CAD build for the part. Positions are in the model's coordinates, mm. Give positions to 0.01 mm unless a question says otherwise; leave off trailing zeros. Loops run counter-clockwise (first coordinate to the right, second up) from the corner with the lowest first, then second, coordinate; pieces in that order, holes last. Notation, with made-up numbers: M 13,27.25 L 53,27.25 A26 ccw 53,52.25 Z; hole C -37,-9 d2. An arc over 180 degrees is marked long. Answer as CSV lines item,"result".
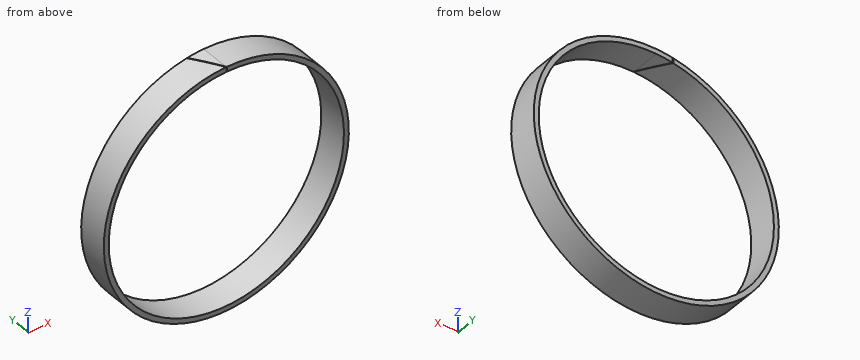
```python
from build123d import *

# Parameters (mm, degrees)
SKETCH1_R           = 25
SKETCH1_R_2         = 24
BOSS_EXTRUDE1_DEPTH = 6
CUT_EXTRUDE1_REACH  = 37.861


with BuildPart() as part:
    # Sketch1 → Boss-Extrude1 (new body)
    with BuildSketch(Plane(origin=(0, 0, 0), x_dir=(1, 0, 0), z_dir=(0, 1, 0))):
        with Locations(Location((0, 0, 0), (0, 0, 270))):
            Circle(SKETCH1_R)
        with Locations(Location((0, 0, 0), (0, 0, 270))):
            Circle(SKETCH1_R_2, mode=Mode.SUBTRACT)
    extrude(amount=BOSS_EXTRUDE1_DEPTH)

    # Sketch2 → Cut-Extrude1 (cut, up to next)
    with BuildSketch(Plane.XY, mode=Mode.PRIVATE) as cut_extrude1_sk1:
        Polygon((0, 0), (-3.464101615, 6), (-3.348631561, 6), (0.115470054, 0), align=None)
    cut_extrude1_tool1 = extrude(cut_extrude1_sk1.sketch, amount=CUT_EXTRUDE1_REACH, mode=Mode.PRIVATE) & part.part
    add(cut_extrude1_tool1.solids().sort_by_distance((-1.674316, 3, 0))[0], mode=Mode.SUBTRACT)


solid = part.part
```
Q1. Wall check: line 1 (Z direction, x = 0, y = 2.75); line 2 (Z direction, x = 6, y = 5.5). Give the ranges that are in metal, low to high. Write a range as [from, to].
Solution:
line 1,"z = [-25, -24], [24, 25]"
line 2,"z = [-24.27, -23.24], [23.24, 24.27]"
Q2. Cut at C-C (y = 4). Write the cut outline in (x, z), and give its area (3 significant figures).
Solution:
outline,"M -2.31,23.89 L -2.31,24.89 A25 ccw long -2.19,24.9 L -2.19,23.9 A24 cw long Z"
area,"154 mm²"
Q3. Pin check, flat tips, straight feed: P1, Ø3, axis at x = 16, y = 3.5, coming from the +Z side; P2, Ø6, axis at x = 15.5, z = 9.5, coming from the +Y side. Stop position of each tip, or through.
Solution:
P1,"stops at z = 20.37"
P2,"passes through"
Q4. Cut at A-A (z = 0). Write the cut outline in (x, y).
Solution:
outline,"M -25,0 L -24,0 L -24,6 L -25,6 Z; M 24,0 L 25,0 L 25,6 L 24,6 Z"
Q5. Cut at B-B (x = 4). Write the cut outline in (y, z), and give its area (3 significant figures).
Solution:
outline,"M 0,-24.68 L 6,-24.68 L 6,-23.66 L 0,-23.66 Z; M 0,23.66 L 6,23.66 L 6,24.68 L 0,24.68 Z"
area,"12.2 mm²"
